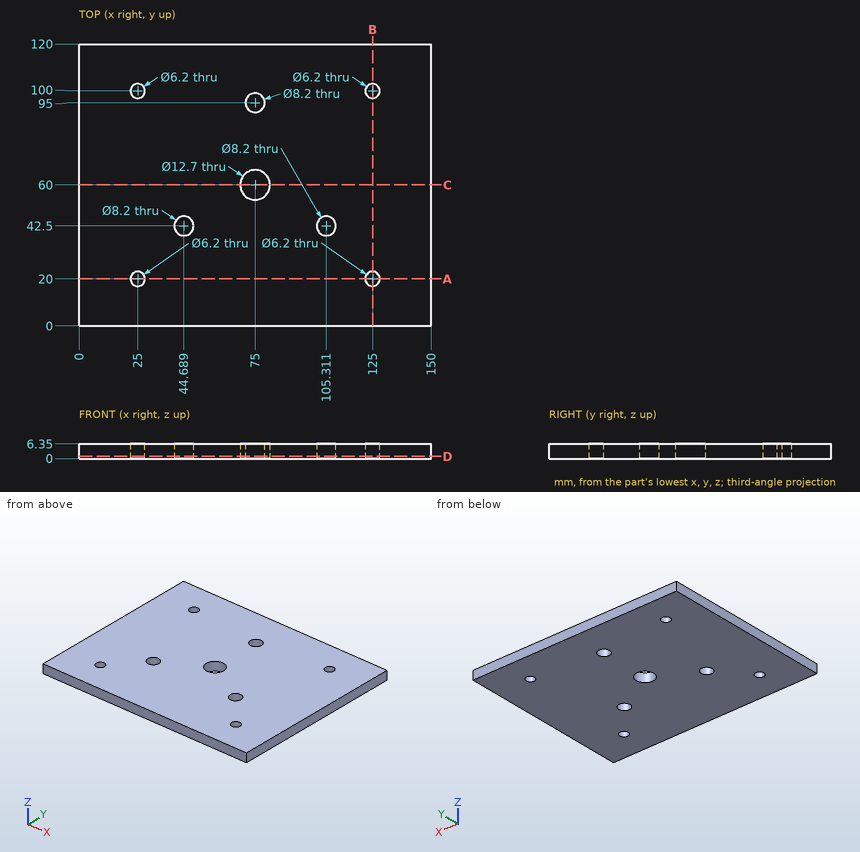
Design review of the part shown in the three views and the two pictorial views. Dimensions are in mm from the part's minimum x, y and z. Round coordinates to 2 decimals unless told otherwise and drop trailing zeros. Loops run counter-clockwise (first coordinate to the right, second up) from the corner with the lowest first, then second, coordinate; pieces in that order, holes last. Notation, with made-up numbers: (84.5, 46) - (126.5, 46) arc R23 ccw to (126.5, 72) - close; hole circle Ø1 at (23, 25.5). An arc over 180 degrees is marked (long way). Write each question's results on one line, items separated by ' | '. Start each with the question number.
Q1. Take a section at A-A on y = 20. Give the boundary of the cut face in (x, z), plus the area to 3 significant figures.
Q2. Wall thickness on line 1 along Y through (x, z) = (75, 2.75); line 2 along Y through (x, z) = (25, 3); line 3 along X through (y, z) = (65, 4) (1 decimal): over which ranges is each line inside the solid? List them lowest first. Write a range as [from, to].
Q3. Take a section at D-D on z = 1. Give the number of separate pieces and of enclosed holes in the cut face, plus the area to 3 significant figures.
Q4. Take a section at B-B on x = 125. Give the boundary of the cut face in (y, z).
Q5. Insertion check: P1, Ø10.5, axis at x = 44.69, y = 42.5, coming from the +Z side. The pin has a flat end and moves straight along its axis. Give the tip position at first contact, or say it passes through.
Q6. Take a section at C-C on y = 60. Give the boundary of the cut face in (x, z), plus the area to 3 significant figures.
Data:
1) outline: (0, 0) - (21.9, 0) - (21.9, 6.35) - (0, 6.35) - close; (28.1, 0) - (121.9, 0) - (121.9, 6.35) - (28.1, 6.35) - close; (128.1, 0) - (150, 0) - (150, 6.35) - (128.1, 6.35) - close | area: 874 mm²
2) line 1: y = [0, 53.65], [66.35, 90.9], [99.1, 120] | line 2: y = [0, 16.9], [23.1, 96.9], [103.1, 120] | line 3: x = [0, 71.1], [78.9, 150]
3) separate pieces: 1 | enclosed holes: 8 | area: 17,600 mm²
4) outline: (0, 0) - (16.9, 0) - (16.9, 6.35) - (0, 6.35) - close; (23.1, 0) - (96.9, 0) - (96.9, 6.35) - (23.1, 6.35) - close; (103.1, 0) - (120, 0) - (120, 6.35) - (103.1, 6.35) - close
5) P1: stops at z = 6.35
6) outline: (0, 0) - (68.65, 0) - (68.65, 6.35) - (0, 6.35) - close; (81.35, 0) - (150, 0) - (150, 6.35) - (81.35, 6.35) - close | area: 872 mm²
